```python
from build123d import *

# Parameters (mm, degrees)
F0_W     = 600
F0_H     = 380
F0_W_2   = 550
F0_H_2   = 152.5
F0_H_3   = 25
F1_DEPTH = 50
F2_DEPTH = 400
F3_DEPTH = 50.001
F4_DEPTH = 400


with BuildPart() as f1:
    # F0 (on Front) → F1 (new body)
    with BuildSketch(Plane.XZ):
        with Locations((300, 190)):
            Rectangle(F0_W, F0_H)
        Polygon((25, 202.5), (25, 355), (575, 355), (575, 202.5), (575, 177.5), (575, 25), (25, 25), (25, 177.5), align=None, mode=Mode.SUBTRACT)
        with Locations((300, 278.75)):
            Rectangle(F0_W_2, F0_H_2)
        with Locations((300, 190)):
            Rectangle(F0_W_2, F0_H_3)
        with Locations((300, 101.25)):
            Rectangle(F0_W_2, F0_H_2)
    extrude(amount=F1_DEPTH)

    # F0 (on Front) → F2 (join)
    with BuildSketch(Plane.XZ):
        with Locations((300, 190)):
            Rectangle(F0_W, F0_H)
        Polygon((25, 202.5), (25, 355), (575, 355), (575, 202.5), (575, 177.5), (575, 25), (25, 25), (25, 177.5), align=None, mode=Mode.SUBTRACT)
    extrude(amount=F2_DEPTH)

    # F3 (cut, through all): a face of the model
    f3_faces = [f1.faces().sort_by_distance(p)[0] for p in [
        (300, -50, 190),
    ]]
    extrude(f3_faces, amount=-F3_DEPTH, mode=Mode.SUBTRACT)

    # F0 (on Front) → F4 (join, through all)
    with BuildSketch(Plane.XZ):
        with Locations((300, 190)):
            Rectangle(F0_W_2, F0_H_3)
    extrude(amount=F4_DEPTH)


solid = f1.part
```
Can you work these out from the model? Positions are in its coordinate system, mm. A direction names the side the tool comes from. Round coordinates to 2 decimals unless told otherwise and drop trailing zeros. Order: outer loops, then holes, each group sorted by start corner. A loop starts at its lowest first (then second) coordinate and runs counter-clockwise, first axis right, second up. Notation, with made-up numbers: (-9.75, -14.75) -> (30.25, -14.75) arc R23 cw to (30.25, -6.75) -> close; hole circle Ø7 at (-30, 28). An arc over 180 degrees is marked (long way). Return JSON: item names as keys, results as strings. Group by question number.
1. If we section it at A-A, the plane x = 407.5: Write out the boundary of the cut face in (y, z), then the cut area to 3 significant figures.
2. If we section it at B-B, the plane z = 330.5: Write out the boundary of the cut face in (x, y), then the cut area to 3 significant figures.
3. I need wall thicknesses on line 1 (Z direction, x = 359, y = -124); line 2 (X direction, y = -52, z = 129.5). Which ranges of each line are inside material? Lowest first, please. Write a range as [from, to].
4. We'd pull the mould along Z, two halves only. Please class faces 1 (the face through (296, -197, 0)), 2 (the face through (296, -197, 380)), 3 (the face through (600, -197, 187)), 4 (the face through (575, -197, 102)): released by +Z, released by -Z, zero draft, split by the parting line, or undercut.
5. If we section it at C-C, the plane y = -162: Write out the boundary of the cut face in (x, z), then the cut area to 4 significant figures.
6. Which directions (+Z, -Z, +X, -X, +Y, -Y) give clear straight access to the entire face, cutting with the end or side of a thin tool? Please do faces 5 (the face through (575, -197, 280)), 6 (the face through (0, -197, 187)).
Output values:
{
 "1": {"outline": "(-400, 0) -> (0, 0) -> (0, 25) -> (-400, 25) -> close; (-400, 177.5) -> (0, 177.5) -> (0, 202.5) -> (-400, 202.5) -> close; (-400, 355) -> (0, 355) -> (0, 380) -> (-400, 380) -> close", "area": "30,000 mm²"},
 "2": {"outline": "(0, -400) -> (25, -400) -> (25, 0) -> (0, 0) -> close; (575, -400) -> (600, -400) -> (600, 0) -> (575, 0) -> close", "area": "20,000 mm²"},
 "3": {"line 1": "[0, 25], [177.5, 202.5], [355, 380]", "line 2": "[0, 25], [575, 600]"},
 "4": {"face 1": "released by -Z", "face 2": "released by +Z", "face 3": "zero draft", "face 4": "undercut"},
 "5": {"outline": "(0, 0) -> (600, 0) -> (600, 380) -> (0, 380) -> close; hole (25, 25) -> (575, 25) -> (575, 177.5) -> (25, 177.5) -> close; hole (25, 202.5) -> (575, 202.5) -> (575, 355) -> (25, 355) -> close", "area": "60,250 mm²"},
 "6": {"face 5": "+Y, -Y", "face 6": "+Z, -Z, -X, +Y, -Y"}
}
